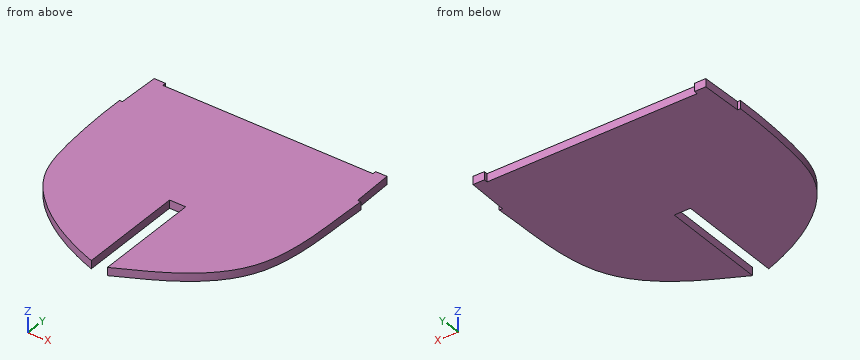
from build123d import *

# Parameters (mm, degrees)
EXTRUDE_1_DEPTH = 4


with BuildPart() as part:
    # 草图1 → 凸台-拉伸1 (new body)
    with BuildSketch(Plane.XY):
        with BuildLine():
            Line((24.544959995, 177.485969069), (128.748328158, 177.485969069))
            Line((128.748328158, 177.485969069), (128.748328158, 179.293294419))
            Line((128.748328158, 179.293294419), (134.346034298, 179.293294419))
            Line((134.346034298, 179.293294419), (134.879857933, 158.745986921))
            Line((134.879857933, 158.745986921), (136.480161375, 158.745986921))
            add(Edge.make_bspline(
                [(82.339222624, 61.799570381), (93.413791621, 67.40108472), (111.733151171, 75.721290264), (128.944446456, 95.047085793), (136.913830684, 122.368393715), (135.612959328, 143.308632698), (136.480161375, 158.745986921)],
                knots=[0, 0, 0, 0, 0.307761121, 0.49025, 0.616329843, 1, 1, 1, 1], degree=3))
            Line((82.339222624, 61.799570381), (82.339222624, 114.477905509))
            Line((82.339222624, 114.477905509), (74.339356348, 114.477905509))
            Line((74.339356348, 114.477905509), (74.339356348, 61.799570381))
            add(Edge.make_bspline(
                [(16.87547225, 158.745986921), (16.656848614, 146.616830277), (17.473837396, 127.05807142), (21.26977179, 98.647925224), (41.890975618, 75.802317121), (61.331956485, 66.364243686), (74.339356348, 61.799570381)],
                knots=[0, 0, 0, 0, 0.287578734, 0.483998215, 0.66783425, 1, 1, 1, 1], degree=3))
            Line((16.87547225, 158.745986921), (18.310507908, 158.745986921))
            Line((18.310507908, 158.745986921), (18.938336008, 179.293294419))
            Line((18.938336008, 179.293294419), (24.544959995, 179.293294419))
            Line((24.544959995, 179.293294419), (24.544959995, 177.485969069))
        make_face()
    extrude(amount=EXTRUDE_1_DEPTH)


solid = part.part
Design review of the part built by this model. Coordinates are the model's own, in mm. Round coordinates to 2 decimals unless told otherwise and drop trailing zeros. Write each loop counter-clockwise with the first axis right and the second up, starting at its lowest first coordinate (ties: lowest second). Pieces come first, ordered by that corner, then holes.
Item 1: For pin 1 Ø2 at (x, z) = (63, 1) entering from +Y; pin 2 Ø1.5 at (y, z) = (140, 1.5) entering from -X; pin 3 Ø1.4 at (y, z) = (178.5, 1.5) entering from +X, all flat-tipped, find the tip position at first contact; note any pin that passes through.
Item 2: Consider section A-A on x = 80.5. Give the boundary of the cut face in (y, z), and give its area (3 significant figures).
Item 3: Consider section B-B on y = 168.5. Give the boundary of the cut face in (x, z), and give its area (3 significant figures).
Item 4: Wall thickness on L1, parallel to Y at x = 79, z = 2.5; L2, parallel to X at y = 106.5, z = 2.9; L3, parallel to X at y = 67, z = 3.6: over which ranges is each line inside the solid? List them lowest first.
Check values:
1. pin 1: stops at y = 177.49
1. pin 2: stops at x = 17.08
1. pin 3: stops at x = 134.38
2. outline: (114.48, 0) - (177.49, 0) - (177.49, 4) - (114.48, 4) - close
2. area: 252 mm2
3. outline: (18.61, 0) - (134.63, 0) - (134.63, 4) - (18.61, 4) - close
3. area: 464 mm2
4. L1: y = 114.48 to 177.49
4. L2: x = 21.01 to 74.34, 82.34 to 132.12
4. L3: x = 61.37 to 74.34, 82.34 to 92.71
